The listing builds one solid part. Answer for the finished solid, in the listing's coordinates (mm). Face numbers are marked on the shaded views. A direction names the side the tool comes from. Round coordinates to 2 decimals unless told otherwise and drop trailing zeros. Write each loop counter-clockwise with the first axis right and the second up, starting at its lowest first coordinate (ties: lowest second). Pieces come first, ordered by that corner, then holes. Notation, with made-up numbers: M 66,30.5 L 83,30.5 A18 ccw 83,51.5 Z; hole C 73,56 d11. An arc over 180 degrees is marked long. Put each result on its own line as item: value. Start each with the question number.
```python
from build123d import *

# Parameters (mm, degrees)
SKETCH1_R           = 4
BOSS_EXTRUDE1_DEPTH = 7
SKETCH2_R           = 3.9
BOSS_EXTRUDE2_DEPTH = 16
CHAMFER1_SIZE       = 0.5
SKETCH3_W           = 3
SKETCH3_H           = 7.2
BOSS_EXTRUDE3_DEPTH = 9


with BuildPart() as part:
    # Sketch1 → Boss-Extrude1 (new body)
    with BuildSketch(Plane(origin=(0, 0, 0), x_dir=(1, 0, 0), z_dir=(0, 1, 0))):
        with Locations(Location((0, 0, 0), (0, 0, 270))):
            Circle(SKETCH1_R)
    extrude(amount=BOSS_EXTRUDE1_DEPTH)

    # Sketch2 → Boss-Extrude2 (add)
    with BuildSketch(Plane(origin=(0, 7, 0), x_dir=(1, 0, 0), z_dir=(0, 1, 0))):
        with Locations(Location((-0.75, 0, 0), (0, 0, 92.228731213))):
            Circle(SKETCH2_R)
    extrude(amount=BOSS_EXTRUDE2_DEPTH)

    # Chamfer1
    chamfer1_edges = [part.edges().sort_by_distance(p)[0] for p in [
        (0, 0, -4),
    ]]
    chamfer(chamfer1_edges, length=CHAMFER1_SIZE)

    # Sketch3 → Boss-Extrude3 (add)
    with BuildSketch(Plane(origin=(0, 23, 0), x_dir=(1, 0, 0), z_dir=(0, 1, 0))):
        with Locations((-0.75, 0)):
            Rectangle(SKETCH3_W, SKETCH3_H)
    extrude(amount=BOSS_EXTRUDE3_DEPTH)


solid = part.part
```
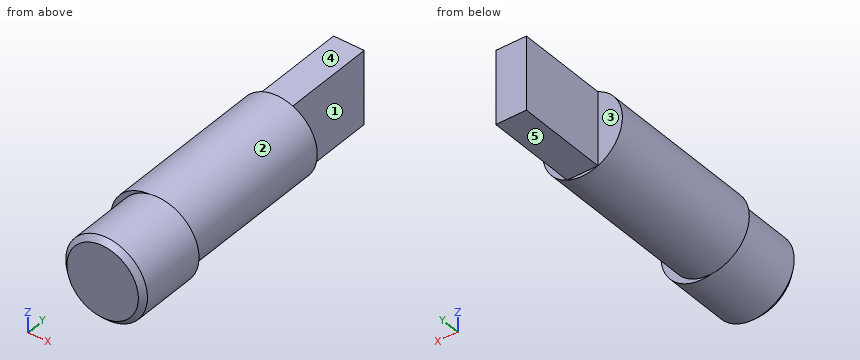
Item 1: Section A-A (z = 0) is taken. Give the vertices of the cut face in (x, y).
Item 2: Flat-ended cylindrical pins translate along their axes: pin 1 (1.5 mm diameter, centred on x = -1.5, z = 1.5, fed in from -Y); pin 2 (3.5 mm diameter, centred on x = -0.5, y = 29, fed in from -Z); pin 3 (2.5 mm diameter, centred on x = -1.5, y = 26.5, fed in from +Z); pin 4 (4 mm diameter, centred on x = 1.5, y = 18.5, fed in from -Z). Find the tip coordinate at first contact, or state that the pin passes through.
Item 3: Section C-C (x = 0) is taken. Give the vertices of the cut face in (y, z), and give its area (3 significant figures).
Item 4: Section B-B (y = 4.5) is taken. Give the vertices of the cut face in (x, z).
Item 5: Which of the six approach directions +Z, -Z, +X, -X, +Y, -Y give full straight-line access (tool end or side, diameter ignored) to the marked faces 1, 2, 3, 4 and 5?
Item 6: Section D-D (y = 23.5) is taken. Give the vertices of the cut face in (x, z), and give its area (3 significant figures).
Item 7: Consider line 1 along Y through (x, z) = (1.5, 2); line 2 along Z through (x, y) = (0.5, 27); line 3 along X through (y, z) = (29.5, -3.5). Determine where each line is inside the solid, lowest interval first. Write a range as [from, to].
Output values:
1. outline: M -4.65,7 L -4,7 L -4,0.5 L -3.5,0 L 3.5,0 L 4,0.5 L 4,7 L 3.15,7 L 3.15,23 L 0.75,23 L 0.75,32 L -2.25,32 L -2.25,23 L -4.65,23 Z
2. pin 1: stops at y = 0
2. pin 2: stops at z = -3.6
2. pin 3: stops at z = 3.6
2. pin 4: stops at z = -3.89
3. outline: M 0,-3.5 L 0.5,-4 L 7,-4 L 7,-3.83 L 23,-3.83 L 23,-3.6 L 32,-3.6 L 32,3.6 L 23,3.6 L 23,3.83 L 7,3.83 L 7,4 L 0.5,4 L 0,3.5 Z
3. area: 243 mm^2
4. outline: C 0,0 d8
5. face 1: +Z, -Z, +X, +Y
5. face 2: +Y
5. face 3: +Z, -Z, -X, +Y
5. face 4: +Z, +X, -X, +Y
5. face 5: -Z, +X, -X, +Y
6. outline: M -2.25,-3.6 L 0.75,-3.6 L 0.75,3.6 L -2.25,3.6 Z
6. area: 21.6 mm^2
7. line 1: y = [0, 23]
7. line 2: z = [-3.6, 3.6]
7. line 3: x = [-2.25, 0.75]
